Job drawing, mm, ordinate dimensions from the low corner. One solid piece. A direction names the side the tool comes from. Coordinates: 2 decimals unless noted, no trailing zeros. Write each loop counter-clockwise with the first axis right and the second up, starting at its lowest first coordinate (ties: lowest second). Pieces come first, ordered by that corner, then holes. Notation, with made-up numbers: (67.5, 85) -> (124.5, 85) arc R27 ccw to (124.5, 109) -> close; hole circle Ø6 at (-35, 70). An arc over 180 degrees is marked (long way). Answer as a JSON object with one key per item and string values. Group by question number.
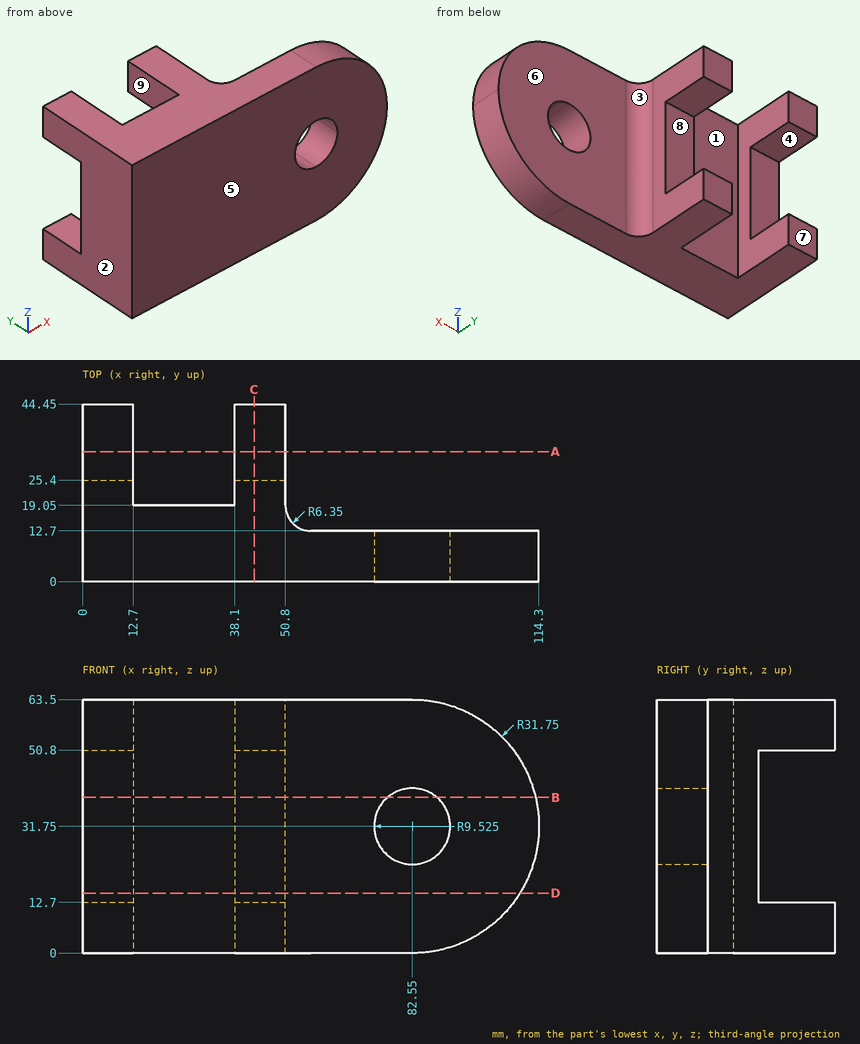
(1) Cut at B-B on z = 39. List the corners of the cut face in (x, y).
(2) Pin check, flat tips, straight feed: pin 1 (12 mm diameter, centred on y = 25, z = 46.5, fed in from +X); pin 2 (2 mm diameter, centred on x = 71.5, z = 30, fed in from +Y); pin 3 (10 mm diameter, centred on x = 6.5, z = 28.5, fed in from +Y). Stop position of each tip, or through.
(3) Cut at C-C on x = 43. List the corners of the cut face in (y, z).
(4) Cut at A-A on y = 32.5. List the corners of the cut face in (x, z).
(5) Wall check: probe 1 along X at (y, z) = (42, 9.5); probe 2 along Z at (x, y) = (50, 28); probe 3 along Y at (x, z) = (101, 35). Give the ranges that are in metal, low to high.
(6) Pull direction X, two halves, no side cores. Call the marked faces 1, 2, 3 and 4: released by +X, released by -X, zero draft, split by the parting line, or undercut.
(7) 3-axis set-ups, long thin cutter, end or side, ignore diameter. For the marked faces 5, 6, 7, 8 and 9: which of +Z, -Z, +X, -X, +Y, -Y reach the whole face in a straight line?
(8) Cut at D-D on z = 15. List the corners of the cut face in (x, y), plus the area to 3 significant figures.
Results found:
{
 "1": {"outline": "(0, 0) -> (76.37, 0) -> (76.37, 12.7) -> (57.15, 12.7) arc R6.35 cw to (50.8, 19.05) -> (50.8, 25.4) -> (38.1, 25.4) -> (38.1, 19.05) -> (12.7, 19.05) -> (12.7, 25.4) -> (0, 25.4) -> close; (88.73, 0) -> (113.46, 0) -> (113.46, 12.7) -> (88.73, 12.7) -> close"},
 "2": {"pin 1": "stops at x = 50.8", "pin 2": "stops at y = 12.7", "pin 3": "stops at y = 25.4"},
 "3": {"outline": "(0, 0) -> (44.45, 0) -> (44.45, 12.7) -> (25.4, 12.7) -> (25.4, 50.8) -> (44.45, 50.8) -> (44.45, 63.5) -> (0, 63.5) -> close"},
 "4": {"outline": "(0, 0) -> (12.7, 0) -> (12.7, 12.7) -> (0, 12.7) -> close; (0, 50.8) -> (12.7, 50.8) -> (12.7, 63.5) -> (0, 63.5) -> close; (38.1, 0) -> (50.8, 0) -> (50.8, 12.7) -> (38.1, 12.7) -> close; (38.1, 50.8) -> (50.8, 50.8) -> (50.8, 63.5) -> (38.1, 63.5) -> close"},
 "5": {"probe 1": "x = 0 to 12.7, 38.1 to 50.8", "probe 2": "z = 0 to 12.7, 50.8 to 63.5", "probe 3": "y = 0 to 12.7"},
 "6": {"face 1": "undercut", "face 2": "released by -X", "face 3": "released by +X", "face 4": "zero draft"},
 "7": {"face 5": "+Z, -Z, +X, -X, -Y", "face 6": "+Z, -Z, +X, +Y", "face 7": "+Z, -Z, +X, -X, +Y", "face 8": "+X, -X, +Y", "face 9": "+Z, -Z, +Y"},
 "8": {"outline": "(0, 0) -> (109.52, 0) -> (109.52, 12.7) -> (57.15, 12.7) arc R6.35 cw to (50.8, 19.05) -> (50.8, 25.4) -> (38.1, 25.4) -> (38.1, 19.05) -> (12.7, 19.05) -> (12.7, 25.4) -> (0, 25.4) -> close", "area": "1,880 mm²"}
}
